Geometry: see drawing. Coordinates: mm, zero at the bounding-box minimum. A direction names the side the tool comes from. Round coordinates to 2 decimals unless told otherwise and drop trailing zeros. Order: outer loops, then holes, each group sorted by start corner. A loop starts at its lowest first (then second) coordinate and runs counter-clockwise, first axis right, second up.
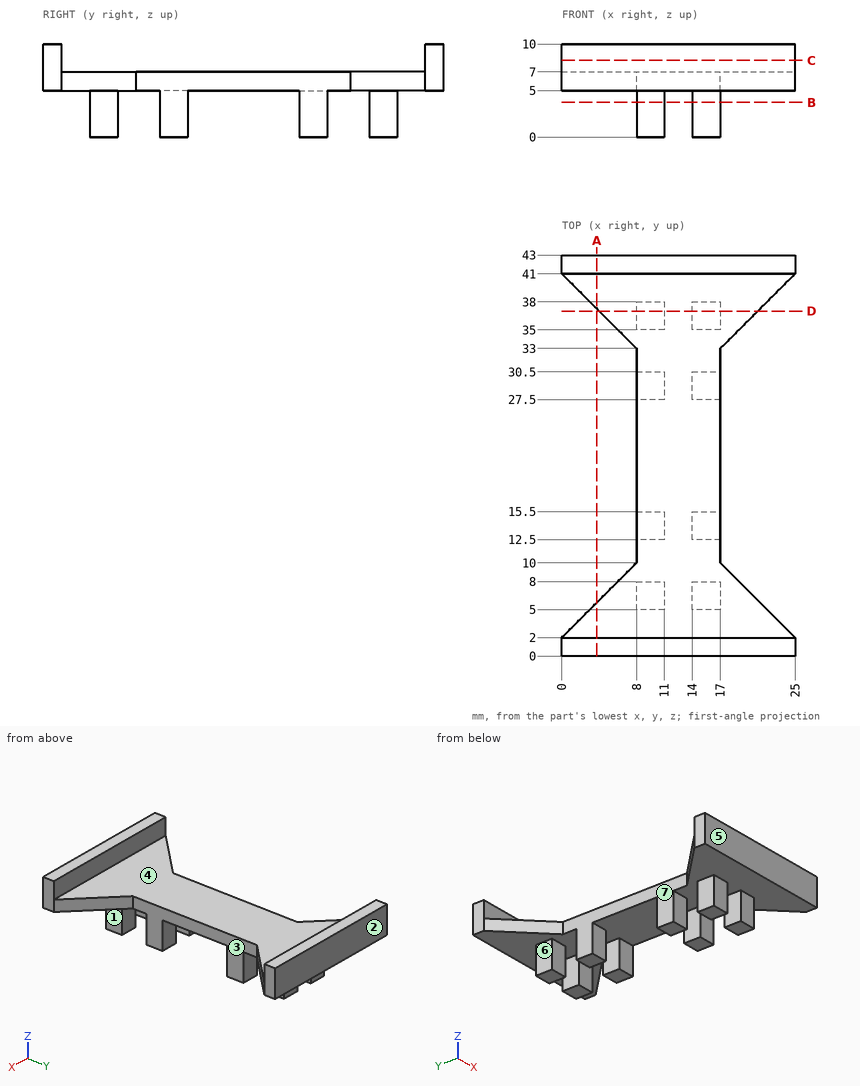
1. Line query: line 1 along Y through (x, z) = (15, 1); line 2 along Y through (x, z) = (4.25, 7.25); line 3 along X through (y, z) = (37.5, 3). Output: solid intervals per line, ascending.
2. First-contact query: pin 1 (2.5 mm diameter, centred on y = 6.5, z = 2, fed in from +X); pin 2 (1.5 mm diameter, centred on x = 16, z = 1.5, fed in from -Y); pin 3 (2.5 mm diameter, centred on x = 9, z = 2, fed in from +Y). Flat tips, straight axial feed; report the tip coordinate or a pass-through.
3. Section B-B on z = 3.75. State how many separate pieces and enclosed holes the cut face has, plus the area to 3 significant figures.
4. Section C-C on z = 8.25. Return loops of the section in (x, y), plus the area to 3 significant figures.
5. Access query for the marked faces 5, 6 and 7. Directions: +Z, -Z, +X, -X, +Y, -Y. A direction counts if a zero-diameter tool reaches every point of the face in a straight line with its end or side. Return the directions, or none.
6. Pull-direction query (Y, two-part tool) for the marked faces 1, 2, 3 and 4; classes: released by +Y, released by -Y, zero draft, split by the parting line, or undercut.
7. Section A-A on x = 3.75. Return loops of the section in (y, z), plus the area to 3 significant figures.
8. Section D-D on y = 37. Return loops of the section in (x, z).
Result:
1. line 1: y = 5 to 8, 12.5 to 15.5, 27.5 to 30.5, 35 to 38
1. line 2: y = 0 to 2, 41 to 43
1. line 3: x = 8 to 11, 14 to 17
2. pin 1: stops at x = 17
2. pin 2: stops at y = 5
2. pin 3: stops at y = 38
3. separate pieces: 8
3. enclosed holes: 0
3. area: 72.0 mm2
4. outline: (0, 0) - (25, 0) - (25, 2) - (0, 2) - close; (0, 41) - (25, 41) - (25, 43) - (0, 43) - close
4. area: 100 mm2
5. face 5: +Z, -Z, +X, -X, -Y
5. face 6: -Z, -X, +Y, -Y
5. face 7: +Z, -Z, -X
6. face 1: zero draft
6. face 2: released by +Y
6. face 3: undercut
6. face 4: undercut
7. outline: (0, 5) - (5.75, 5) - (5.75, 7) - (2, 7) - (2, 10) - (0, 10) - close; (37.25, 5) - (43, 5) - (43, 10) - (41, 10) - (41, 7) - (37.25, 7) - close
7. area: 35.0 mm2
8. outline: (4, 5) - (8, 5) - (8, 0) - (11, 0) - (11, 5) - (14, 5) - (14, 0) - (17, 0) - (17, 5) - (21, 5) - (21, 7) - (4, 7) - close
